from build123d import *

# Parameters (mm, degrees)
F0_W     = 42.4481438452
F0_H     = 2
F1_DEPTH = 3
F2_DEPTH = 10
F3_R     = 1.5
F4_R     = 1
F5_R     = 3
F6_R     = 5


with BuildPart() as f1:
    # F0 (on Top) → F1 (new body)
    with BuildSketch(Plane.XY):
        Polygon((-65.7136544558, 49.5634722376), (-65.7136544558, 36.4734722376), (-65.7136544558, 35.0634722376), (-65.7136544558, 33.6534722376), (-65.7136544558, 20.5634722376), (-7.7136544558, 18.5634722376), (-7.7136544558, 51.5634722376), align=None)
        with Locations((-36.7136544558, 32.6534722376)):
            Rectangle(F0_W, F0_H, mode=Mode.SUBTRACT)
        with Locations((-36.7136544558, 37.4734722376)):
            Rectangle(F0_W, F0_H, mode=Mode.SUBTRACT)
    extrude(amount=F1_DEPTH)

    # F0 (on Top) → F2 (join)
    with BuildSketch(Plane.XY):
        with Locations((-36.7136544558, 32.6534722376)):
            Rectangle(F0_W, F0_H)
        with Locations((-36.7136544558, 37.4734722376)):
            Rectangle(F0_W, F0_H)
    extrude(amount=F2_DEPTH)

    # F3
    f3_edges = [f1.edges().sort_by_distance(p)[0] for p in [
        (-57.937726, 36.473472, 6.5),
        (-57.937726, 33.653472, 6.5),
        (-15.489583, 36.473472, 6.5),
        (-15.489583, 33.653472, 6.5),
    ]]
    fillet(f3_edges, radius=F3_R)

    # F4
    f4_edges = [f1.edges().sort_by_distance(p)[0] for p in [
        (-36.713654, 36.473472, 10),
        (-36.713654, 33.653472, 10),
        (-57.498387, 33.214132, 10),
        (-15.928922, 33.214132, 10),
        (-57.937726, 31.903472, 10),
        (-15.489583, 31.903472, 10),
        (-57.937726, 38.223472, 10),
        (-57.498387, 36.912812, 10),
        (-15.489583, 38.223472, 10),
        (-15.928922, 36.912812, 10),
    ]]
    fillet(f4_edges, radius=F4_R)

    # F5
    f5_edges = [f1.edges().sort_by_distance(p)[0] for p in [
        (-7.713654, 18.563472, 1.5),
        (-7.713654, 51.563472, 1.5),
    ]]
    fillet(f5_edges, radius=F5_R)

    # F6
    f6_edges = [f1.edges().sort_by_distance(p)[0] for p in [
        (-65.713654, 20.563472, 1.5),
        (-65.713654, 49.563472, 1.5),
    ]]
    fillet(f6_edges, radius=F6_R)


solid = f1.part
Can you work these out from the model? Positions are in its coordinate system, mm. A direction names the side the tool comes from. Coordinates: 2 decimals unless noted, no trailing zeros. Write each loop counter-clockwise with the first axis right and the second up, starting at its lowest first coordinate (ties: lowest second). Pieces come first, ordered by that corner, then holes. Notation, with made-up numbers: (49, -10.75) -> (103, -10.75) arc R22 ccw to (103, 8.25) -> close; hole circle Ø7 at (23.25, 78). An arc over 180 degrees is marked (long way). Answer as CSV lines item,"result".
1) If we section it at D-D on x = -55: Please give me the cut outline in (y, z).
Check result:
outline,"(20.19, 0) -> (49.93, 0) -> (49.93, 3) -> (38.47, 3) -> (38.47, 10) -> (37.47, 10) arc R1 ccw to (36.47, 9) -> (36.47, 3) -> (33.65, 3) -> (33.65, 9) arc R1 ccw to (32.65, 10) -> (31.65, 10) -> (31.65, 3) -> (20.19, 3) -> close"
2) If we section it at A-A on z = 7.25: Please give me the cut outline in (x, y), then the cut area to 3 significant figures.
Check result:
outline,"(-57.94, 31.65) -> (-15.49, 31.65) -> (-15.49, 32.15) arc R1.5 ccw to (-16.99, 33.65) -> (-56.44, 33.65) arc R1.5 ccw to (-57.94, 32.15) -> close; (-57.94, 37.97) arc R1.5 ccw to (-56.44, 36.47) -> (-16.99, 36.47) arc R1.5 ccw to (-15.49, 37.97) -> (-15.49, 38.47) -> (-57.94, 38.47) -> close"
area,"168 mm²"
3) On a 3-axis mill with a long thin cutter (end or side, diameter ignored), from which of +Z, -Z, +X, -X, +Y, -Y can I reach the whole of each face in a straight line? I mean faces 1 (the cylindrical face through (-15.941, 33.226, 6.042)), 2 (the flat face through (-37, 31.653, 6)), 3 (the cylindrical face through (-57.51, 33.2, 6.04)), 4 (the flat face through (-37, 38.473, 6)), 5 (the flat face through (-37, 36.473, 6)). Say none if no direction works.
Check result:
face 1,"+Z, +X"
face 2,"+Z, +X, -X, -Y"
face 3,"+Z, -X"
face 4,"+Z, +X, -X, +Y"
face 5,"+Z, +X, -X"
4) If we section it at C-C on x = -26: Please give me the cut outline in (y, z).
Check result:
outline,"(19.19, 0) -> (50.93, 0) -> (50.93, 3) -> (38.47, 3) -> (38.47, 10) -> (37.47, 10) arc R1 ccw to (36.47, 9) -> (36.47, 3) -> (33.65, 3) -> (33.65, 9) arc R1 ccw to (32.65, 10) -> (31.65, 10) -> (31.65, 3) -> (19.19, 3) -> close"
5) Will these pins go through, and if not, where does the flat tip stop? P1, Ø3, axis at x = -41, z = 5, coming from the +Y side; P2, Ø5, axis at x = -30.5, z = 7, coming from the -Y side; P3, Ø1.5, axis at x = -14, y = 26, coming from the +Z side.
Check result:
P1,"y = 38.47"
P2,"y = 31.65"
P3,"z = 3"
6) If we section it at B-B on z = 1: Please give me the cut outline in (x, y).
Check result:
outline,"(-65.71, 25.39) arc R5 ccw to (-60.89, 20.4) -> (-10.82, 18.67) arc R3 ccw to (-7.71, 21.67) -> (-7.71, 48.46) arc R3 ccw to (-10.82, 51.46) -> (-60.89, 49.73) arc R5 ccw to (-65.71, 44.73) -> close"
7) If I drill on line 1 (Y direction, x = -27, z = 8); line 2 (Z direction, x = -43.5, y = 25); line 3 (Y direction, x = -57, z = 6.25), over which ranges is the centre line in solid material (lowest first)? Write a range as from..to.
Check result:
line 1,"31.65..33.65, 36.47..38.47"
line 2,"0..3"
line 3,"31.65..33.54, 36.58..38.47"
